The model under review builds one solid part; all positions refer to its coordinate system, in mm. A direction names the side the tool comes from. Coordinates: 2 decimals unless noted, no trailing zeros. Write each loop counter-clockwise with the first axis right and the second up, starting at its lowest first coordinate (ties: lowest second). Pieces come first, ordered by that corner, then holes. Notation, with made-up numbers: (42, -25.5) - (56, -25.5) arc R19 cw to (56, -19.5) - close; hole circle Ø11 at (18, 3). An arc over 180 degrees is marked (long way). Put each result on its own line as item: value. Start each with the question number.
Item 1: Mouldability with a two-part tool opening along X and no side actions: class faces 4 (the face through (-51.57, 1.97, 51.67)), 5 (the face through (-1, 4, -1)), 6 (the face through (51.67, 1.97, 51.57)), 7 (the face through (-39.966, 1.972, -40.577)) as pulls with the +X half, pulls with the -X half, needs draft (parallel to the pull), parting line crosses it, or undercut.
Item 2: Consider section A-A on y = 1.75. Give the boundary of the cut face in (x, z), then the cut area to 3 significant figures.
Item 3: Consider section B-B on x = 0. Give the boundary of the cut face in (y, z).
Item 4: Machinability: for faces 1 (the face through (0, 2, 40)), 2 (the face through (0, 2, -40)), 3 (the face through (51.57, 1.97, -51.67)), which of the approach directions +Z, -Z, +X, -X, +Y, -Y give a long, thin tool a straight path to every point of the face, cutting with its end or side? Answer none if there is none.
Item 5: To check wall thickness, follow L1, parallel to X at y = 2.45, z = 39; L2, parallel to X at y = 0.45, z = 38; L3, parallel to X at y = 2.55, z = 44. State the ranges of each line that lie inside material, in increasing order. Write a range as [from, to].
Item 6: For pin 1 (2.5 mm diameter, centred on x = -38.89, z = 38.89, fed in from -Y), flat-tipped, find the tip position at first contact; note if it passes through.
```python
from build123d import *

# Parameters (mm, degrees)
BOSS_EXTRUDE1_DEPTH   = 4
F_4_0MM_DOWEL_HOLE2_D = 4
FILLET1_START         = -1
FILLET1_DEPTH         = 6
FILLET1_2_DEPTH       = 4


with BuildPart() as part:
    # Sketch1 → Boss-Extrude1 (new body)
    with BuildSketch(Plane(origin=(0, 0, 0), x_dir=(1, 0, 0), z_dir=(0, 1, 0))):
        with BuildLine():
            Line((55, 48), (55, -48))
            ThreePointArc((55, -48), (51.618795027, -51.618795027), (48, -55))
            Line((48, -55), (17.5, -55))
            Line((17.5, -55), (17.5, -40))
            Line((17.5, -40), (-17.5, -40))
            Line((-17.5, -40), (-17.5, -55))
            Line((-17.5, -55), (-48, -55))
            ThreePointArc((-48, -55), (-51.618795027, -51.618795027), (-55, -48))
            Line((-55, -48), (-55, 48))
            ThreePointArc((-55, 48), (-51.618795027, 51.618795027), (-48, 55))
            Line((-48, 55), (-17.5, 55))
            Line((-17.5, 55), (-17.5, 40))
            Line((-17.5, 40), (17.5, 40))
            Line((17.5, 40), (17.5, 55))
            Line((17.5, 55), (48, 55))
            ThreePointArc((48, 55), (51.618795027, 51.618795027), (55, 48))
        make_face()
    extrude(amount=BOSS_EXTRUDE1_DEPTH)

    # Ø4.0mm Dowel Hole2 (through all)
    with Locations(Plane(origin=(0, 4, 0), x_dir=(1, 0, 0), z_dir=(0, 1, 0))):
        with Locations((38.890872965, 38.890872965), (38.890872965, -38.890872965), (-38.890872965, -38.890872965), (-38.890872965, 38.890872965)):
            Hole(F_4_0MM_DOWEL_HOLE2_D / 2)

    # Fillet1: read off the stored shape, not the designer's step
    # Fillet1 outline → Fillet1 (cut)
    with BuildSketch(Plane(origin=(0, 0, 0), x_dir=(1, 0, 0), z_dir=(0, 1, 0)).offset(FILLET1_START)):
        with BuildLine():
            Line((17.5, 55), (17.5, 47.5))
            ThreePointArc((17.5, 47.5), (19.696699141, 52.803300859), (25, 55))
            Line((25, 55), (17.5, 55))
        make_face()
        with BuildLine():
            ThreePointArc((-25, 55), (-19.696699141, 52.803300859), (-17.5, 47.5))
            Line((-17.5, 47.5), (-17.5, 55))
            Line((-17.5, 55), (-25, 55))
        make_face()
        with BuildLine():
            Line((-17.5, -55), (-17.5, -47.5))
            ThreePointArc((-17.5, -47.5), (-19.696699141, -52.803300859), (-25, -55))
            Line((-25, -55), (-17.5, -55))
        make_face()
        with BuildLine():
            ThreePointArc((25, -55), (19.696699141, -52.803300859), (17.5, -47.5))
            Line((17.5, -47.5), (17.5, -55))
            Line((17.5, -55), (25, -55))
        make_face()
    extrude(amount=FILLET1_DEPTH, mode=Mode.SUBTRACT)

    # Fillet1 2 outline → Fillet1 2 (add)
    with BuildSketch(Plane(origin=(0, 0, 0), x_dir=(1, 0, 0), z_dir=(0, 1, 0))):
        with BuildLine():
            Line((-17.5, 40), (-10, 40))
            ThreePointArc((-10, 40), (-15.303300859, 42.196699141), (-17.5, 47.5))
            Line((-17.5, 47.5), (-17.5, 40))
        make_face()
        with BuildLine():
            ThreePointArc((17.5, 47.5), (15.303300859, 42.196699141), (10, 40))
            Line((10, 40), (17.5, 40))
            Line((17.5, 40), (17.5, 47.5))
        make_face()
        with BuildLine():
            Line((17.5, -40), (10, -40))
            ThreePointArc((10, -40), (15.303300859, -42.196699141), (17.5, -47.5))
            Line((17.5, -47.5), (17.5, -40))
        make_face()
        with BuildLine():
            ThreePointArc((-17.5, -47.5), (-15.303300859, -42.196699141), (-10, -40))
            Line((-10, -40), (-17.5, -40))
            Line((-17.5, -40), (-17.5, -47.5))
        make_face()
    extrude(amount=FILLET1_2_DEPTH)


solid = part.part
```
Report:
1. face 4: pulls with the -X half
1. face 5: needs draft
1. face 6: pulls with the +X half
1. face 7: undercut
2. outline: (-55, -48) arc R73 ccw to (-48, -55) - (-25, -55) arc R7.5 ccw to (-17.5, -47.5) arc R7.5 cw to (-10, -40) - (10, -40) arc R7.5 cw to (17.5, -47.5) arc R7.5 ccw to (25, -55) - (48, -55) arc R73 ccw to (55, -48) - (55, 48) arc R73 ccw to (48, 55) - (25, 55) arc R7.5 ccw to (17.5, 47.5) arc R7.5 cw to (10, 40) - (-10, 40) arc R7.5 cw to (-17.5, 47.5) arc R7.5 ccw to (-25, 55) - (-48, 55) arc R73 ccw to (-55, 48) - close; hole circle Ø4 at (-38.89, -38.89); hole circle Ø4 at (-38.89, 38.89); hole circle Ø4 at (38.89, -38.89); hole circle Ø4 at (38.89, 38.89)
2. area: 10,900 mm²
3. outline: (0, -40) - (4, -40) - (4, 40) - (0, 40) - close
4. face 1: +Z, +Y, -Y
4. face 2: -Z, +Y, -Y
4. face 3: -Z, +X, +Y, -Y
5. L1: [-55, -40.89], [-36.89, 36.89], [40.89, 55]
5. L2: [-55, -40.68], [-37.1, 37.1], [40.68, 55]
5. L3: [-55, -16.63], [16.63, 55]
6. pin 1: through
